CAD build for the part. Positions are in the model's coordinates, mm. A direction names the side the tool comes from. Give positions to 0.01 mm unless a question says otherwise; leave off trailing zeros. Loops run counter-clockwise (first coordinate to the right, second up) from the corner with the lowest first, then second, coordinate; pieces in that order, holes last. Notation, with made-up numbers: M 51,11.5 L 56,11.5 A35 cw 56,49.5 Z; hole C -6,-1 d9. An arc over 180 degrees is marked long. Answer as CSV lines item,"result".
from build123d import *

# Parameters (mm, degrees)
EXTRUDE_1_DEPTH     = 6
SKETCH_2_R          = 1
CUT_EXTRUDE_1_DEPTH = 38.831864876


with BuildPart() as part:
    # 草图1 → 凸台-拉伸1 (new body)
    with BuildSketch(Plane.XY):
        with BuildLine():
            Line((8.215752349, -15.451582875), (23.643338017, -7.248590067))
            ThreePointArc((23.643338017, -7.248590067), (25.005690113, -6.897786494), (26.378171201, -7.206593948))
            Line((26.378171201, -7.206593948), (33, -10.470749302))
            Line((33, -10.470749302), (28.760739296, -0.470749302))
            ThreePointArc((28.760739296, -0.470749302), (16.956768231, 12.637944122), (0, 17.5))
            ThreePointArc((0, 17.5), (-4.233633173, 16.98017521), (-8.215752349, 15.451582875))
            Line((-8.215752349, 15.451582875), (-23.643338017, 7.248590067))
            ThreePointArc((-23.643338017, 7.248590067), (-25.005690113, 6.897786494), (-26.378171201, 7.206593948))
            Line((-26.378171201, 7.206593948), (-33, 10.470749302))
            Line((-33, 10.470749302), (-28.760739296, 0.470749302))
            ThreePointArc((-28.760739296, 0.470749302), (-16.956768231, -12.637944122), (0, -17.5))
            ThreePointArc((0, -17.5), (4.233633173, -16.98017521), (8.215752349, -15.451582875))
        make_face()
        with BuildLine():
            Line((-3, -4), (3, -4))
            ThreePointArc((3, -4), (3.707106781, -3.707106781), (4, -3))
            Line((4, -3), (4, 3))
            ThreePointArc((4, 3), (3.707106781, 3.707106781), (3, 4))
            Line((3, 4), (-3, 4))
            ThreePointArc((-3, 4), (-3.707106781, 3.707106781), (-4, 3))
            Line((-4, 3), (-4, -3))
            ThreePointArc((-4, -3), (-3.707106781, -3.707106781), (-3, -4))
        make_face(mode=Mode.SUBTRACT)
    extrude(amount=EXTRUDE_1_DEPTH)

    # 草图2 → 切除-拉伸1 (cut, through all)
    with BuildSketch(Plane.XY.offset(6)):
        with Locations((0, 10)):
            Circle(SKETCH_2_R)
        with Locations((7.071067812, 7.071067812)):
            Circle(SKETCH_2_R)
        with Locations((10, 0)):
            Circle(SKETCH_2_R)
        with Locations((7.071067812, -7.071067812)):
            Circle(SKETCH_2_R)
        with Locations((0, -10)):
            Circle(SKETCH_2_R)
        with Locations((-7.071067812, -7.071067812)):
            Circle(SKETCH_2_R)
        with Locations((-10, 0)):
            Circle(SKETCH_2_R)
        with Locations((-7.071067812, 7.071067812)):
            Circle(SKETCH_2_R)
    extrude(amount=-CUT_EXTRUDE_1_DEPTH, mode=Mode.SUBTRACT)


solid = part.part
1) Drill centre lines: line 1 (Y direction, x = 1.5, z = 5.85); line 2 (Y direction, x = 10, z = 2.65); line 3 (Y direction, x = 13, z = 3.75). Where is each one in solid material? Low to high. Write a range as from..to.
Answer below:
line 1,"y = -17.44..-4, 4..17.46"
line 2,"y = -14.5..-1, 1..15.9"
line 3,"y = -12.91..14.74"
2) Flat gauge pins, fed straight in: pin 1 (1.6 mm diameter, centred on x = 7.07, y = -7.07, fed in from +Z); pin 2 (1.8 mm diameter, centred on y = 0, z = 2, fed in from -X); pin 3 (1.8 mm diameter, centred on y = -1, z = 2.5, fed in from +X). Where does each tip first touch, or does it go through?
Answer below:
pin 1,"passes through"
pin 2,"stops at x = -28.94"
pin 3,"stops at x = 29.37"
3) Band-saw the part on B-B on z = 1.4. Give the number of separate pieces and of enclosed holes in the cut face, and give its area (3 significant figures).
Answer below:
separate pieces,"1"
enclosed holes,"9"
area,"1,360 mm^2"
4) Mould opens along X. For faces 1 (the face through (-15.82, 11.41, 2.96)), 2 (the face through (17.168, 12.505, 2.958)), 3 (the face through (-30.91, 5.54, 2.96)) say: +X half, -X half, draft (parallel to the pull), parting line (faces both ways), or undercut.
Answer below:
face 1,"undercut"
face 2,"+X half"
face 3,"-X half"
5) Which spindle directions (+Z, -Z, +X, -X, +Y, -Y) get a long thin tool onto all of the face, cutting with end or side? Do faces 4 (the face through (0, 4, 3)), 5 (the face through (7, 0, 0)), 6 (the face through (29.643, -8.816, 2.958)). Say none if no direction does.
Answer below:
face 4,"+Z, -Z"
face 5,"-Z, +X, -X, +Y, -Y"
face 6,"+Z, -Z, -Y"
6) Band-saw the part on D-D on y = -12. Give the cut face in (x, z), and give its area (3 significant figures).
Answer below:
outline,"M -17.94,0 L 14.71,0 L 14.71,6 L -17.94,6 Z"
area,"196 mm^2"
7) Band-saw the part on A-A on x = -10. Give the cut face in (y, z), and give its area (3 significant figures).
Answer below:
outline,"M -15.9,0 L -1,0 L -1,6 L -15.9,6 Z; M 1,0 L 14.5,0 L 14.5,6 L 1,6 Z"
area,"170 mm^2"
8) Band-saw the part on C-C on x = -2. Give the cut face in (y, z).
Answer below:
outline,"M -17.44,0 L -4,0 L -4,6 L -17.44,6 Z; M 4,0 L 17.39,0 L 17.39,6 L 4,6 Z"
